Autodesk Fusion 360 part; units mm, degrees
sketch "Sketch1" plane through (0, 0, 0) normal (0, 0, 1) x (1, 0, 0)
  circle A0 centre (0, 0) radius 50
extrude "Extrude1" add sketch "Sketch1" along normal blind 400
sketch "Sketch2" plane through (0, 0, 400) normal (0, 0, 1) x (-1, 0, 0)
  circle A0 centre (0, 0) radius 50
  line L0 (-28, -3) -> (-19.7737, -3)
  line L1 (-19.7737, 3) -> (-28, 3)
  line L2 (-28, 3) -> (-28, -3)
  arc A1 (-19.7737, -3) -> (-19.7737, 3) centre (0, 0) ccw
extrude "Extrude2" add sketch "Sketch2" along normal blind 110 contours L0 L1 L2 A1
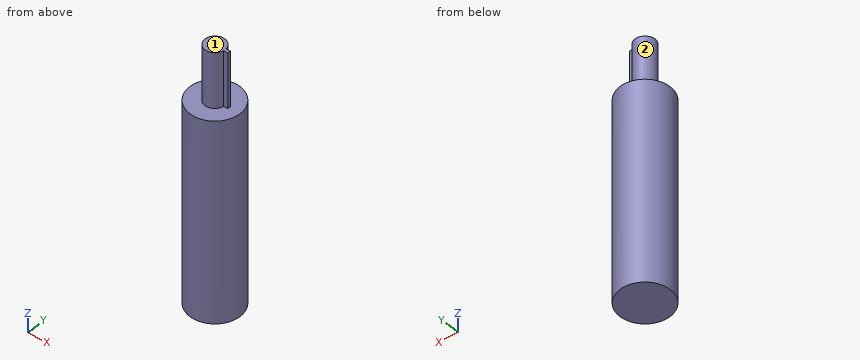
Can you work these out from the model? Positions are in its coordinate system, mm. Face numbers are marked on the shaded views. A direction names the side the tool comes from. Coordinates: 2 decimals unless noted, no trailing zeros. Loops run counter-clockwise (first coordinate to the right, second up) from the corner with the lowest first, then second, coordinate; pieces in that order, holes last. Notation, with made-up numbers: M 71,17 L 114,17 A28 cw 114,39 Z; hole C 1,45.5 d1. An arc over 180 degrees is marked long. Put each result on its own line as item: value. Start each with the question number.
(1) Imagine slicing it at B-B on y = 12.5. List the corners of the cut face in (x, z) for me.
(2) Imagine slicing it at D-D on x = -27.5. List the corners of the cut face in (y, z) for me.
(3) Imagine slicing it at C-C on z = 425.5. List the corners of the cut face in (x, y) for me.
(4) Which directions (+Z, -Z, +X, -X, +Y, -Y) give clear straight access to the entire face, cutting with the end or side of a thin tool? Please do the marked faces 1 and 2.
(5) Will these pins go through, and if not, where does the flat tip stop? pin 1 Ø6 at (y, z) = (5.5, 80.5) entering from +X; pin 2 Ø1 at (y, z) = (-14.5, 152) entering from +X; pin 3 Ø4 at (x, z) = (26, 455.5) entering from -Y.
(6) I need wall thicknesses on probe 1 along Z at (x, y) = (-12, -22); probe 2 along Y at (x, z) = (38, 206); probe 3 along Y at (x, z) = (-4, 422). Which ranges of each line are inside material? Lowest first, please.
(7) Imagine slicing it at A-A on x = 0. List the corners of the cut face in (y, z) for me.
Worked answers:
1. outline: M -48.41,0 L 48.41,0 L 48.41,400 L 15.61,400 L 15.61,510 L -15.61,510 L -15.61,400 L -48.41,400 Z
2. outline: M -41.76,0 L 41.76,0 L 41.76,400 L -41.76,400 Z
3. outline: M 19.77,-3 L 28,-3 L 28,3 L 19.77,3 A20 ccw long Z
4. face 1: +Z, +X, -X, +Y, -Y
4. face 2: +Z
5. pin 1: stops at x = 49.94
5. pin 2: stops at x = 48
5. pin 3: stops at y = -3
6. probe 1: z = 0 to 400
6. probe 2: y = -32.5 to 32.5
6. probe 3: y = -19.6 to 19.6
7. outline: M -50,0 L 50,0 L 50,400 L 20,400 L 20,510 L -20,510 L -20,400 L -50,400 Z
